Verification items for the finished model (mm, model axes). A direction names the side the tool comes from. Give positions to 0.01 mm unless a question says otherwise; leave off trailing zeros. Write each loop counter-clockwise with the first axis right and the second up, starting at its lowest first coordinate (ties: lowest second). Pieces come first, ordered by that corner, then holes.
from build123d import *

# Parameters (mm, degrees)
F0_W         = 28
F0_H         = 18
F1_DEPTH     = 3
F2_DEPTH     = 25
F3_R         = 2
F4_R         = 1
F5_DEPTH     = 50
F0_W_2       = 2.2
F0_H_2       = 4.5
F6_DEPTH     = 10
F9_DEPTH     = 100
F4_R_2       = 3.125
F10_R        = 3.125
F10_R_2      = 1
F11_DEPTH    = 0.75
F12_T1_DEPTH = 25.6433879336
F12_T3_DEPTH = 13.1433879336
F12_T5_DEPTH = 15.5
F13_DEPTH    = 35
F14_DEPTH    = 39
F15_T1_DEPTH = 28
F7_R         = 2
F7_R_2       = 1
F8_R         = 2
F8_R_2       = 1
F16_DEPTH    = 1.5


# Not quite as in the source:
# - a fillet or chamfer that OpenCascade refuses, or shapes differently, is made with other operations: its cross-section is extruded or revolved along the edge and cut away or added


with BuildPart() as f1:
    # F0 (on Top) → F1 (new body)
    with BuildSketch(Plane.XY):
        Polygon((-17.5, 0), (-17.5, -7), (-13.5, -7), (-13.5, 0), (-13.5, 1), (-14, 1), (-16.2, 1), (-16.2, 5.5), (-14, 5.5), (-14, 13), (-14, 31), (-17.5, 31), align=None)
        Polygon((-13.5, 0), (-13.5, -7), (13.5, -7), (13.5, 0), (12.5, 0), (12.5, -4), (0.5, -4), (0.5, 0), align=None)
        Polygon((13.5, 0), (13.5, -7), (17.5, -7), (17.5, 0), (17.5, 31), (14, 31), (14, 13), (14, 5.5), (16.2, 5.5), (16.2, 1), (14, 1), (13.5, 1), align=None)
        with Locations((0, 22)):
            Rectangle(F0_W, F0_H)
    extrude(amount=F1_DEPTH)

    # F0 (on Top) → F2 (join)
    with BuildSketch(Plane.XY):
        Polygon((-17.5, 0), (-17.5, -7), (-13.5, -7), (-13.5, 0), (-13.5, 1), (-14, 1), (-16.2, 1), (-16.2, 5.5), (-14, 5.5), (-14, 13), (-14, 31), (-17.5, 31), align=None)
        Polygon((13.5, 0), (13.5, -7), (17.5, -7), (17.5, 0), (17.5, 31), (14, 31), (14, 13), (14, 5.5), (16.2, 5.5), (16.2, 1), (14, 1), (13.5, 1), align=None)
    extrude(amount=F2_DEPTH)

    # F3
    f3_edges = [f1.edges().sort_by_distance(p)[0] for p in [
        (0, 13, 3),
        (6.5, -4, 3),
    ]]
    fillet(f3_edges, radius=F3_R)

    # F4 (on face) → F5 (cut, symmetric)
    with BuildSketch(Plane(origin=(13.5, 0, 0), x_dir=(0, -1, 0), z_dir=(-1, 0, 0))):
        with Locations((3.8, 17)):
            Circle(F4_R)
    extrude(amount=F5_DEPTH, both=True, mode=Mode.SUBTRACT)

    # F0 (on Top) → F6 (join)
    with BuildSketch(Plane.XY):
        with Locations((15.1, 3.25)):
            Rectangle(F0_W_2, F0_H_2)
        with Locations((-15.1, 3.25)):
            Rectangle(F0_W_2, F0_H_2)
    extrude(amount=F6_DEPTH)

    # F7 (on face) → F9 (cut)
    with BuildSketch(Plane(origin=(-17.5, 0, 0), x_dir=(0, -1, 0), z_dir=(-1, 0, 0))):
        Polygon((-31, 25), (-31, 3), (-30.5205184888, 3), (-30.311506, 3.940513), (-30.015185, 5.062344), (-29.67651, 6.184174), (-29.274339, 7.284839), (-28.829835, 8.364339), (-28.343022, 9.422672), (-27.792668, 10.459839), (-27.200003, 11.475841), (-26.565008, 12.470677), (-25.88768, 13.402016), (-25.146834, 14.333332), (-24.384844, 15.222339), (-23.580522, 16.069015), (-22.755012, 16.894503), (-21.887171, 17.67768), (-20.97702, 18.418505), (-20.066847, 19.138164), (-19.114343, 19.815513), (-18.119507, 20.450509), (-17.124671, 21.064339), (-16.108669, 21.657003), (-15.071502, 22.207335), (-14.034334, 22.736502), (-12.976001, 23.244503), (-11.896502, 23.710172), (-10.817003, 24.154675), (-9.737503, 24.556847), (-8.636839, 24.958997), (-8.5183879336, 25), align=None)
    extrude(amount=-F9_DEPTH, mode=Mode.SUBTRACT)

    # F4 (on face) + F10 (on face) → F11 (cut, symmetric)
    with BuildSketch(Plane(origin=(13.5, 0, 0), x_dir=(0, -1, 0), z_dir=(-1, 0, 0))):
        with Locations((3.8, 17)):
            Circle(F4_R_2)
        with Locations((3.8, 17)):
            Circle(F4_R, mode=Mode.SUBTRACT)
    with BuildSketch(Plane.YZ.offset(-13.5)):
        with Locations((-3.8, 17)):
            Circle(F10_R)
        with Locations((-3.8, 17)):
            Circle(F10_R_2, mode=Mode.SUBTRACT)
    extrude(amount=F11_DEPTH, both=True, dir=(-1, 0, 0), mode=Mode.SUBTRACT)

    # F12: fillet of radius 1.5 on 6 edges, made by hand

    # F12_s2 → F12_t1 (cut)
    with BuildSketch(Plane.XZ.offset(-14.8933879336)):
        with BuildLine():
            ThreePointArc((16, 25), (17.0606601718, 24.5606601718), (17.5, 23.5))
            Line((17.5, 23.5), (17.5, 25))
            Line((17.5, 25), (16, 25))
        make_face()
        with BuildLine():
            ThreePointArc((-17.5, 23.5), (-17.0606601718, 24.5606601718), (-16, 25))
            Line((-16, 25), (-17.5, 25))
            Line((-17.5, 25), (-17.5, 23.5))
        make_face()
    extrude(amount=F12_T1_DEPTH, mode=Mode.SUBTRACT)

    # F12_s4 → F12_t3 (cut)
    with BuildSketch(Plane.XZ.offset(-14.8933879336)):
        with BuildLine():
            ThreePointArc((15.5, 25), (14.4393398282, 24.5606601718), (14, 23.5))
            Line((14, 23.5), (14, 25))
            Line((14, 25), (15.5, 25))
        make_face()
        with BuildLine():
            ThreePointArc((-14, 23.5), (-14.4393398282, 24.5606601718), (-15.5, 25))
            Line((-15.5, 25), (-14, 25))
            Line((-14, 25), (-14, 23.5))
        make_face()
    extrude(amount=F12_T3_DEPTH, mode=Mode.SUBTRACT)

    # F12_s6 → F12_t5 (cut)
    with BuildSketch(Plane.XZ.offset(-4.75)):
        with BuildLine():
            ThreePointArc((13.5, 23.5), (13.9393398282, 24.5606601718), (15, 25))
            Line((15, 25), (13.5, 25))
            Line((13.5, 25), (13.5, 23.5))
        make_face()
        with BuildLine():
            ThreePointArc((-13.5, 23.5), (-13.9393398282, 24.5606601718), (-15, 25))
            Line((-15, 25), (-13.5, 25))
            Line((-13.5, 25), (-13.5, 23.5))
        make_face()
    extrude(amount=F12_T5_DEPTH, mode=Mode.SUBTRACT)

    # F7 (on face) → F13 (join)
    with BuildSketch(Plane(origin=(-17.5, 0, 0), x_dir=(0, -1, 0), z_dir=(-1, 0, 0))):
        Polygon((-30.311506, 3.940513), (-30.5205184888, 3), (-28.0815777779, 3), (-28.0815777779, 5.062344), (-30.015185, 5.062344), align=None)
    extrude(amount=-F13_DEPTH)

    # F7 (on face) → F14 (cut)
    with BuildSketch(Plane(origin=(-17.5, 0, 0), x_dir=(0, -1, 0), z_dir=(-1, 0, 0))):
        Polygon((-31, 3), (-31, 0), (-30.946502, 0.490336), (-30.777175, 1.654498), (-30.565517, 2.797516), (-30.5205184888, 3), align=None)
    extrude(amount=-F14_DEPTH, mode=Mode.SUBTRACT)

    # F15: fillet of radius 2 on 1 edges, made by hand

    # F15_s2 → F15_t1 (cut)
    with BuildSketch(Plane.YZ.offset(-14)):
        with BuildLine():
            ThreePointArc((28.0815777779, 3.063446304), (28.6440824638, 4.4539883645), (30.015185, 5.062344))
            Line((30.015185, 5.062344), (28.0815777779, 5.062344))
            Line((28.0815777779, 5.062344), (28.0815777779, 3.063446304))
        make_face()
    extrude(amount=F15_T1_DEPTH, mode=Mode.SUBTRACT)

    # F7 (on face) + F8 (on face) → F16 (cut, symmetric)
    with BuildSketch(Plane(origin=(-17.5, 0, 0), x_dir=(0, -1, 0), z_dir=(-1, 0, 0))):
        with Locations((3.8, 17)):
            Circle(F7_R)
        with Locations((3.8, 17)):
            Circle(F7_R_2, mode=Mode.SUBTRACT)
    with BuildSketch(Plane.YZ.offset(17.5)):
        with Locations((-3.8, 17)):
            Circle(F8_R)
        with Locations((-3.8, 17)):
            Circle(F8_R_2, mode=Mode.SUBTRACT)
    extrude(amount=F16_DEPTH, both=True, dir=(-1, 0, 0), mode=Mode.SUBTRACT)


solid = f1.part
Item 1: Sectioned sample at A-A on y = 7. Record the cut outline in (x, z).
Answer key:
outline: (-17.5, 0) - (-14, 0) - (-14, 23.5) arc R1.5 ccw to (-15.5, 25) - (-16, 25) arc R1.5 ccw to (-17.5, 23.5) - close; (14, 0) - (17.5, 0) - (17.5, 23.5) arc R1.5 ccw to (16, 25) - (15.5, 25) arc R1.5 ccw to (14, 23.5) - close
Item 2: Scan lines: line 1 along X through (y, z) = (5.5, 4.25); line 2 along X through (y, z) = (-3.5, 7.75); line 3 along Z through (x, y) = (13, -3). Record each from-to range of solid material in increasing order.
Answer key:
line 1: x = -17.5 to -14, 14 to 17.5
line 2: x = -17.5 to -13.5, 13.5 to 17.5
line 3: z = 0 to 3
Item 3: Release check for a two-part mould opening along X. For faces 5 (the face through (15.725, 25.522, 13.861)), 6 (the face through (-14.262, 8.225, 24.347)), 7 (the face through (-16, -3, 18)), 8 (the face through (15, 3, 10)) record: released by +X, released by -X, zero draft, split by the parting line, or undercut.
Answer key:
face 5: zero draft
face 6: undercut
face 7: released by -X
face 8: undercut
Item 4: Set-up check for faces 1 (the face through (-16.2, 3, 17)), 2 (the face through (-13.9, -4.2, 20.1)), 3 (the face through (13.93, -2.94, 24.55)), 4 (the face through (-6, 0, 1)): record each of +Z, -Z, +X, -X, +Y, -Y from which the full face is reachable in a straight line by a thin tool's end or side.
Answer key:
face 1: +Z
face 2: none
face 3: +Z, +Y, -Y
face 4: +Z, -Z
Item 5: Sectioned sample at B-B on x = 5. Record the cut outline in (y, z), then the cut area to 3 significant figures.
Answer key:
outline: (-7, 0) - (-4, 0) - (-4, 1) arc R2 ccw to (-6, 3) - (-7, 3) - close; (13, 0) - (31, 0) - (30.95, 0.49) - (30.78, 1.65) - (30.57, 2.8) - (30.31, 3.94) - (30.02, 5.06) arc R2 ccw to (28.08, 3.06) - (28.08, 3) - (15, 3) arc R2 ccw to (13, 1) - close
area: 64.3 mm2
Item 6: Depth check by flat-ended pin: pin 1 (3.5 mm diameter, centred on y = -3.8, z = 17, fed in from -X); pin 2 (1 mm diameter, centred on x = 11.5, z = 2.5, fed in from +Y); pin 3 (2 mm diameter, centred on x = 10.5, y = 21, fed in from +Z); pin 4 (1.2 mm diameter, centred on y = -3.8, z = 17, fed in from -X). Enter the tip coordinate at first touch or a pass-through.
Answer key:
pin 1: stops at x = -16
pin 2: stops at y = 30.71
pin 3: stops at z = 3
pin 4: passes through
Item 7: Sectioned sample at C-C on x = -13. Record the cut outline in (y, z).
Answer key:
outline: (-7, 0) - (0, 0) - (0, 3) - (-7, 3) - close; (13, 0) - (31, 0) - (30.95, 0.49) - (30.78, 1.65) - (30.57, 2.8) - (30.31, 3.94) - (30.02, 5.06) arc R2 ccw to (28.08, 3.06) - (28.08, 3) - (15, 3) arc R2 ccw to (13, 1) - close
